```python
from build123d import *

# Parameters (mm, degrees)
SKETCH_1_W      = 3
SKETCH_1_H      = 15
EXTRUDE_1_DEPTH = 3


with BuildPart() as part:
    # 草图1 → 凸台-拉伸1 (new body)
    with BuildSketch(Plane.XY):
        Polygon((20, 0), (180, 0), (180, -3), (200, -3), (200, 0), (202.75, 0), (207.75, 0), (207.75, 30), (202.75, 30), (200, 30), (0, 30), (-2.75, 30), (-7.75, 30), (-7.75, 0), (-2.75, 0), (0, 0), (0, -3), (20, -3), align=None)
        with Locations((204.25, 15)):
            Rectangle(SKETCH_1_W, SKETCH_1_H, mode=Mode.SUBTRACT)
        with Locations((-4.25, 15)):
            Rectangle(SKETCH_1_W, SKETCH_1_H, mode=Mode.SUBTRACT)
        Polygon((100, 5), (105, 5), (105, 20), (95, 20), (95, 5), align=None, mode=Mode.SUBTRACT)
    extrude(amount=EXTRUDE_1_DEPTH)


solid = part.part
```
The listing builds one solid part. Answer for the finished solid, in the listing's coordinates (mm). Give positions to 0.01 mm unless a question says otherwise; leave off trailing zeros. Loops run counter-clockwise (first coordinate to the right, second up) from the corner with the lowest first, then second, coordinate; pieces in that order, holes last. Notation, with made-up numbers: M -9,69 L 33,69 A32 ccw 33,97 Z; hole C -15,6.25 d6. An arc over 180 degrees is marked long. One line per item, written item: value.
Q1. Find the intervals of material crossed by line 1 (X direction, y = 11.5, z = 0.5); line 2 (X direction, y = 7, z = 1.4); line 3 (Y direction, x = 100, z = 0.8), in increasing order. Write a range as from..to.
Working result:
line 1: x = -7.75..-5.75, -2.75..95, 105..202.75, 205.75..207.75
line 2: x = -7.75..95, 105..207.75
line 3: y = 0..5, 20..30
Q2. Flat-ended cylindrical pins translate along their axes: P1, Ø1.5, axis at x = -4, z = 1.5, coming from the -Y side; P2, Ø1, axis at x = 103.5, y = 15.5, coming from the -Z side; P3, Ø0.9, axis at y = -1.5, z = 2, coming from the -X side. Find the tip coordinate at first contact, or state that the pin passes through.
Working result:
P1: stops at y = 0
P2: passes through
P3: stops at x = 0
Q3. A cutting plane is placed at D-D on x = 152.5. Determine the outline of the cut face in (y, z), then the cut area to 3 significant figures.
Working result:
outline: M 0,0 L 30,0 L 30,3 L 0,3 Z
area: 90.0 mm^2
Q4. A cutting plane is placed at B-B on x = 101.5. Determine the outline of the cut face in (y, z), then the cut area to 3 significant figures.
Working result:
outline: M 0,0 L 5,0 L 5,3 L 0,3 Z; M 20,0 L 30,0 L 30,3 L 20,3 Z
area: 45.0 mm^2
Q5. A cutting plane is placed at A-A on y = 17.5. Determine the outline of the cut face in (x, z).
Working result:
outline: M -7.75,0 L -5.75,0 L -5.75,3 L -7.75,3 Z; M -2.75,0 L 95,0 L 95,3 L -2.75,3 Z; M 105,0 L 202.75,0 L 202.75,3 L 105,3 Z; M 205.75,0 L 207.75,0 L 207.75,3 L 205.75,3 Z
Q6. A cutting plane is placed at C-C on z = 1.65. Determine the outline of the cut face in (x, y).
Working result:
outline: M -7.75,0 L 0,0 L 0,-3 L 20,-3 L 20,0 L 180,0 L 180,-3 L 200,-3 L 200,0 L 207.75,0 L 207.75,30 L -7.75,30 Z; hole M -5.75,7.5 L -2.75,7.5 L -2.75,22.5 L -5.75,22.5 Z; hole M 95,5 L 105,5 L 105,20 L 95,20 Z; hole M 202.75,7.5 L 205.75,7.5 L 205.75,22.5 L 202.75,22.5 Z
